from build123d import *

# Parameters (mm, degrees)
SKETCH1_R           = 1.85
BOSS_EXTRUDE1_DEPTH = 4.318


with BuildPart() as part:
    # Sketch1 → Boss-Extrude1 (new body)
    with BuildSketch(Plane(origin=(0, 0, 0), x_dir=(0, 0, -1), z_dir=(1, 0, 0))):
        with BuildLine():
            Line((136.240741284, 32.272255751), (136.240741284, 82.154119676))
            ThreePointArc((136.240741284, 82.154119676), (111.765249408, 180.544448903), (44.044009042, 256))
            Line((44.044009042, 256), (-215.955990958, 256))
            ThreePointArc((-215.955990958, 256), (-271.683097829, 163.39777941), (-296.50139881, 58.208741794))
            ThreePointArc((-296.50139881, 58.208741794), (-295.198004633, 52.399053051), (-290.863193916, 48.3172966))
            Line((-290.863193916, 48.3172966), (-257.759258716, 32))
            Line((-257.759258716, 32), (-257.759258716, 5))
            ThreePointArc((-257.759258716, 5), (-256.294792622, 1.464466094), (-252.759258716, 0))
            Line((-252.759258716, 0), (-231.380747369, 0))
            ThreePointArc((-231.380747369, 0), (-175.759258716, 37.5), (-120.137770063, 0))
            Line((-120.137770063, 0), (40.619252631, 0))
            ThreePointArc((40.619252631, 0), (78.000395352, 34.660211514), (128.548433592, 28.059005308))
            ThreePointArc((128.548433592, 28.059005308), (133.642663591, 27.886965654), (136.240741284, 32.272255751))
        make_face()
        with Locations((-207.955990958, 48)):
            Circle(SKETCH1_R, mode=Mode.SUBTRACT)
        with Locations((-191.955990958, 48)):
            Circle(SKETCH1_R, mode=Mode.SUBTRACT)
        with Locations((-199.955990958, 40)):
            Circle(SKETCH1_R, mode=Mode.SUBTRACT)
        with Locations((-199.955990958, 200)):
            Circle(SKETCH1_R, mode=Mode.SUBTRACT)
        with Locations((-191.955990958, 240)):
            Circle(SKETCH1_R, mode=Mode.SUBTRACT)
        with Locations((-207.955990958, 240)):
            Circle(SKETCH1_R, mode=Mode.SUBTRACT)
        with Locations((-199.955990958, 248)):
            Circle(SKETCH1_R, mode=Mode.SUBTRACT)
        with Locations((-199.955990958, 88)):
            Circle(SKETCH1_R, mode=Mode.SUBTRACT)
        with Locations((-111.759258716, 16)):
            Circle(SKETCH1_R, mode=Mode.SUBTRACT)
        with Locations((32.240741284, 16)):
            Circle(SKETCH1_R, mode=Mode.SUBTRACT)
        with Locations((24.240741284, 8)):
            Circle(SKETCH1_R, mode=Mode.SUBTRACT)
        with Locations((-103.759258716, 8)):
            Circle(SKETCH1_R, mode=Mode.SUBTRACT)
        with Locations((-28.820215612, 192.5)):
            Circle(SKETCH1_R, mode=Mode.SUBTRACT)
        with Locations((-20.820215612, 200.5)):
            Circle(SKETCH1_R, mode=Mode.SUBTRACT)
        with Locations((-28.820215612, 208.5)):
            Circle(SKETCH1_R, mode=Mode.SUBTRACT)
        with Locations((26.544009042, 238)):
            Circle(SKETCH1_R, mode=Mode.SUBTRACT)
        with Locations((10.544009042, 238)):
            Circle(SKETCH1_R, mode=Mode.SUBTRACT)
        with Locations((18.544009042, 246)):
            Circle(SKETCH1_R, mode=Mode.SUBTRACT)
        Polygon((-93.121069237, 82.721950219), (-81.186806492, 81.46760866), (-81.680426507, 76.771127937), (-93.614689252, 78.025469496), align=None, mode=Mode.SUBTRACT)
        Polygon((-35.639064197, 76.680348038), (-23.704801453, 75.426006479), (-24.198421467, 70.729525756), (-36.132684212, 71.983867315), align=None, mode=Mode.SUBTRACT)
    extrude(amount=BOSS_EXTRUDE1_DEPTH)


solid = part.part
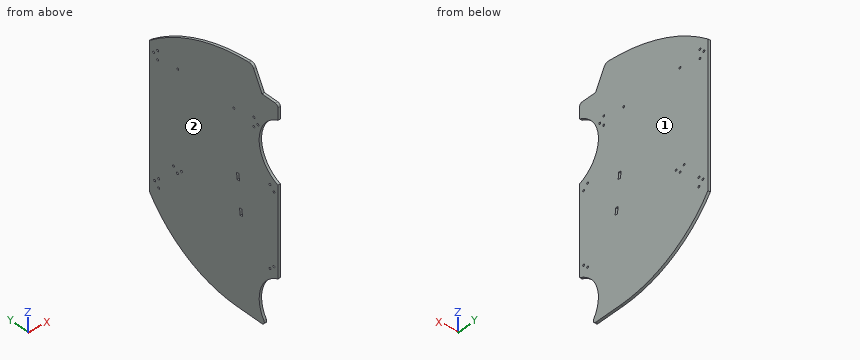
The listing builds one solid part. Answer for the finished solid, in the listing's coordinates (mm). Face numbers are marked on the shaded views. Give positions to 0.01 mm unless a question says otherwise; leave off trailing zeros. Loops run counter-clockwise (first coordinate to the right, second up) from the corner with the lowest first, then second, coordinate; pieces in that order, holes last.
Item 1: Determine the mould class of the marked faces 1 and 2 for opening direction X: +X half, -X half, draft (parallel to the pull), parting line (faces both ways), or undercut.
Derived:
face 1: +X half
face 2: -X half
Item 2: Each of these flat-tipped pins is pushed along its axis until it touches: pin 1 Ø2 at (y, z) = (200.5, 20.82) entering from -X; pin 2 Ø2 at (x, z) = (3.5, 154.5) entering from -Y. Where does it stop, or does it pass through?
Derived:
pin 1: passes through
pin 2: stops at y = 33.22
Item 3: Find the intervals of material crossed by line 1 along Z through (x, y) = (3, 56.5); line 2 along Z through (x, y) = (2.7, 240); line 3 along Z through (x, y) = (3.3, 248), in increasing order.
Derived:
line 1: z = -136.24 to 296.49
line 2: z = -64.75 to 190.11, 193.81 to 206.11, 209.81 to 228.57
line 3: z = -55.06 to 198.11, 201.81 to 222.45
Item 4: A cutting plane is placed at A-A (y = 127.5). Give the vertices of the cut face in (x, z).
Derived:
outline: (0, -131.29) - (4.32, -131.29) - (4.32, 284.08) - (0, 284.08) - close
Item 5: A cutting plane is placed at C-C (z = 183). Give the vertices of the cut face in (x, y), then the cut area to 3 significant figures.
Derived:
outline: (0, 37.06) - (4.32, 37.06) - (4.32, 256) - (0, 256) - close
area: 945 mm2
Item 6: A cutting plane is placed at B-B (x = 2). Give the number of separate pieces and of enclosed holes in the cut face, then the cut area to 3 significant figures.
Derived:
separate pieces: 1
enclosed holes: 20
area: 92,700 mm2
